Input: dimensioned drawing with shaded views. Units: mm. Origin: part minimum x, y, z. Round coordinates to 2 decimals unless told otherwise and drop trailing zeros. Order: outer loops, then holes, each group sorted by start corner. A loop starts at its lowest first (then second) coordinate and runs counter-clockwise, first axis right, second up. Notation, with made-up numbers: (-24.5, 69.5) - (10.5, 69.5) arc R19 cw to (10.5, 102.5) - close; hole circle Ø3 at (-16.75, -40). An arc over 180 degrees is marked (long way). Put each result on its own line as item: value. Start each with the question number.
(1) Section B-B (x = 35.5). Output: boundary loops of the cut face in (y, z), and give its area (3 significant figures).
(2) Section D-D (z = 2.5). Output: boundary loops of the cut face in (x, y).
(3) Section A-A (y = 35). Output: boundary loops of the cut face in (x, z).
(4) Section C-C (y = 58.5). Output: boundary loops of the cut face in (x, z).
(5) Material intervals for L1, parallel to Y at x = 35, z = 4; L2, parallel to X at y = 33.5, z = 11; L3, parallel to Y at x = 34, z = 3, sorted ascending. Write a range as [from, to].
(6) Pull-direction query (Y, two-part tool) for the marked faces 1, 2, 3 and 4; classes: released by +Y, released by -Y, zero draft, split by the parting line, or undercut.
(7) Pin query (flat end, axial travel): P1, Ø6, axis at y = 46, z = 5, coming from the +X side; P2, Ø3, axis at x = 30.5, z = 5.5, coming from the +Y side; P3, Ø1.5, axis at x = 32, y = 21, coming from the +Z side. Return the tip coordinate at first contact, or that it passes through.
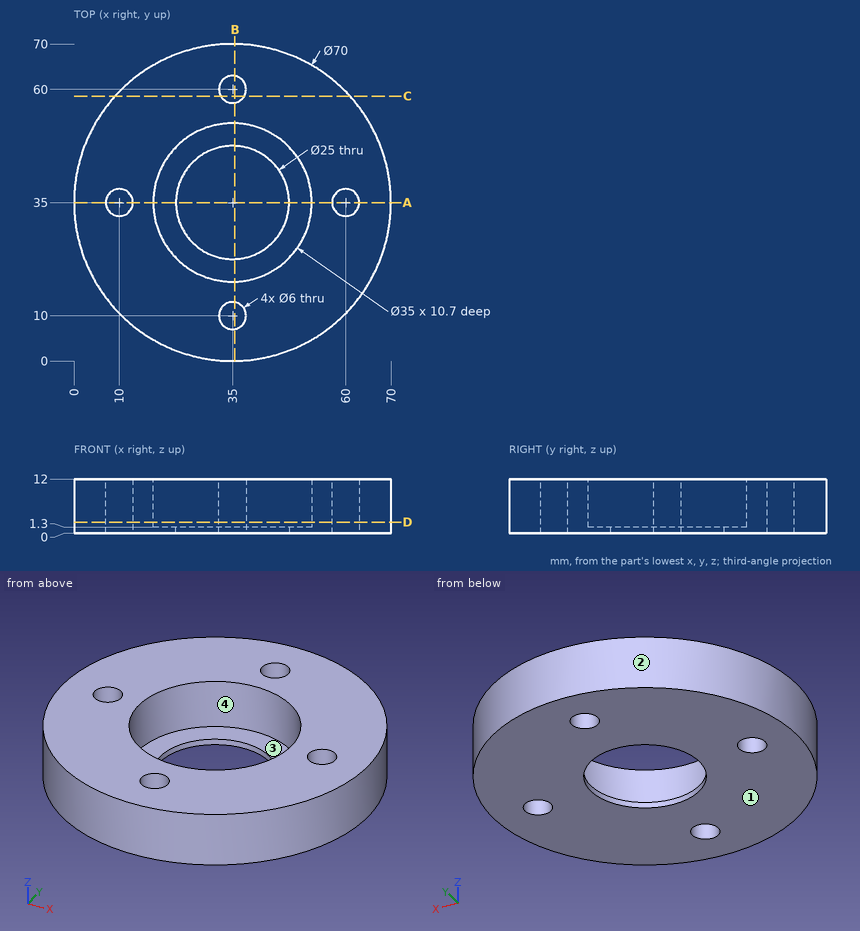
Checks:
1. outline: (0, 0) - (7.04, 0) - (7.04, 12) - (0, 12) - close; (12.96, 0) - (22.51, 0) - (22.51, 1.3) - (17.51, 1.3) - (17.51, 12) - (12.96, 12) - close; (47.49, 0) - (57.04, 0) - (57.04, 12) - (52.49, 12) - (52.49, 1.3) - (47.49, 1.3) - close; (62.96, 0) - (70, 0) - (70, 12) - (62.96, 12) - close
1. area: 291 mm²
2. outline: circle Ø70 at (35, 35); hole circle Ø6 at (10, 35); hole circle Ø35 at (35, 35); hole circle Ø6 at (35, 10); hole circle Ø6 at (35, 60); hole circle Ø6 at (60, 35)
3. outline: (0, 0) - (7, 0) - (7, 12) - (0, 12) - close; (13, 0) - (22.5, 0) - (22.5, 1.3) - (17.5, 1.3) - (17.5, 12) - (13, 12) - close; (47.5, 0) - (57, 0) - (57, 12) - (52.5, 12) - (52.5, 1.3) - (47.5, 1.3) - close; (63, 0) - (70, 0) - (70, 12) - (63, 12) - close
4. outline: (9.06, 0) - (32.4, 0) - (32.4, 12) - (9.06, 12) - close; (37.6, 0) - (60.94, 0) - (60.94, 12) - (37.6, 12) - close
5. L1: y = [0, 7], [13, 17.5], [52.5, 57], [63, 70]
5. L2: x = [0.03, 7.4], [12.6, 17.56], [52.44, 57.4], [62.6, 69.97]
5. L3: y = [0.01, 7.17], [12.83, 17.53], [52.47, 57.17], [62.83, 69.99]
6. face 1: zero draft
6. face 2: split by the parting line
6. face 3: undercut
6. face 4: undercut
7. P1: stops at x = 69.07
7. P2: stops at y = 69.87
7. P3: stops at z = 1.3
